The model under review builds one solid part; all positions refer to its coordinate system, in mm. A direction names the side the tool comes from. Round coordinates to 2 decimals unless told otherwise and drop trailing zeros. Loops run counter-clockwise (first coordinate to the right, second up) from the corner with the lowest first, then second, coordinate; pieces in that order, holes last. Notation, with made-up numbers: (-1, -28.75) - (58, -28.75) arc R29 ccw to (58, -7.75) - close; hole circle Ø7 at (21.25, 15.5). An arc over 180 degrees is marked (long way). Answer as CSV lines item,"result".
from build123d import *

# Parameters (mm, degrees)
F0_R      = 7.9
F0_R_2    = 6.9
F1_DEPTH  = 12
F2_R      = 12.5
F3_DEPTH  = 0.5
F3_FACE_R = 6.9
F4_DEPTH  = 0.5


with BuildPart() as f1:
    # F0 (on Front) → F1 (new body)
    with BuildSketch(Plane.XZ):
        Circle(F0_R)
        Circle(F0_R_2, mode=Mode.SUBTRACT)
    extrude(amount=F1_DEPTH)

    # F2 (on Front) → F3 (join)
    with BuildSketch(Plane.XZ):
        Circle(F2_R)
    extrude(amount=F3_DEPTH)

    # F3_face (on face) → F4 (cut)
    with BuildSketch(Plane.XZ.offset(0.5)):
        Circle(F3_FACE_R)
    extrude(amount=-F4_DEPTH, mode=Mode.SUBTRACT)


solid = f1.part
1. Draft analysis for pull direction Z (two halves, no side actions). For faces 1 (the face through (11.923, -0.246, 3.755)), 2 (the face through (-0.9, -6.08, 6.84)), 3 (the face through (5, 0, -5)), state which applies: +Z half, -Z half, draft (parallel to the pull), parting line (faces both ways), or undercut.
Numbers:
face 1,"parting line"
face 2,"undercut"
face 3,"draft"
2. Take a section at C-C (y = -11). State the section outline as (x, z) points.
Numbers:
outline,"circle Ø15.8 at (0, 0); hole circle Ø13.8 at (0, 0)"
3. Take a section at B-B (x = 0). State the section outline as (y, z) points.
Numbers:
outline,"(-12, -7.9) - (-0.5, -7.9) - (-0.5, -12.5) - (0, -12.5) - (0, -6.9) - (-12, -6.9) - close; (-12, 6.9) - (0, 6.9) - (0, 12.5) - (-0.5, 12.5) - (-0.5, 7.9) - (-12, 7.9) - close"
4. Take a section at D-D (x = 7.5). State the section outline as (y, z) points.
Numbers:
outline,"(-12, -2.48) - (-0.5, -2.48) - (-0.5, -10) - (0, -10) - (0, 10) - (-0.5, 10) - (-0.5, 2.48) - (-12, 2.48) - close"
5. Wall thickness on probe 1 along Z at (x, y) = (0, -6); probe 2 along Y at (x, z) = (-9.25, -1.75); probe 3 along Z at (x, y) = (2.75, -1.75): over which ranges is each line inside the solid? List them lowest first.
Numbers:
probe 1,"z = -7.9 to -6.9, 6.9 to 7.9"
probe 2,"y = -0.5 to 0"
probe 3,"z = -7.41 to -6.33, 6.33 to 7.41"
6. Tool access review of faces 4 (the face through (-0.2, -0.5, -8.2)), 5 (the face through (1, -12, -7)): name each direction out of +Z, -Z, +X, -X, +Y, -Y from which nothing blocks a thin tool from reaching the whole face with its end or side.
Numbers:
face 4,"-Y"
face 5,"+Z, -Z, +X, -X, -Y"
7. Take a section at A-A (z = 0). State the section outline as (x, y) points.
Numbers:
outline,"(-12.5, -0.5) - (-7.9, -0.5) - (-7.9, -12) - (-6.9, -12) - (-6.9, 0) - (-12.5, 0) - close; (6.9, -12) - (7.9, -12) - (7.9, -0.5) - (12.5, -0.5) - (12.5, 0) - (6.9, 0) - close"
8. Clearance check with flat-ended pins moving along their axes: pin 1 (2 mm diameter, centred on x = 1.5, y = -8, fed in from -Z); pin 2 (3 mm diameter, centred on x = 1.5, y = -7, fed in from +Z); pin 3 (12.5 mm diameter, centred on x = -6, z = 1, fed in from -Y); pin 4 (1.5 mm diameter, centred on y = -9, z = 1, fed in from +X). State where each tip first meets the part, or that it passes through.
Numbers:
pin 1,"stops at z = -7.88"
pin 2,"stops at z = 7.9"
pin 3,"stops at y = -12"
pin 4,"stops at x = 7.9"
